from build123d import *

# Parameters (mm, degrees)
F0_W     = 60
F0_H     = 30
F1_DEPTH = 30
F2_W     = 30
F2_H     = 30
F3_DEPTH = 40
F3_TAPER = 7
F4_R     = 5.4270060884
F5_DEPTH = 40


with BuildPart() as f1:
    # F0 (on Front) → F1 (new body)
    with BuildSketch(Plane.XZ):
        with Locations((-30, -15)):
            Rectangle(F0_W, F0_H)
    extrude(amount=F1_DEPTH)

    # F2 (on face) → F3 (join)
    with BuildSketch(Plane.XY):
        with Locations((-15, -15)):
            Rectangle(F2_W, F2_H)
    extrude(amount=F3_DEPTH, taper=F3_TAPER)

    # F4 (on face) → F5 (cut)
    with BuildSketch(Plane.XY.offset(40)):
        with Locations((-14.5341902971, -15)):
            Circle(F4_R)
    extrude(amount=-F5_DEPTH, mode=Mode.SUBTRACT)


solid = f1.part
Geometry check sheet. Reference: the model listing, model coordinates, mm. A direction names the side the tool comes from. Give positions to 0.01 mm unless a question says otherwise; leave off trailing zeros. Order: outer loops, then holes, each group sorted by start corner. A loop starts at its lowest first (then second) coordinate and runs counter-clockwise, first axis right, second up.
1) Cross-section at C-C (x = -3.5). Record the boundary of the cut face in (y, z), then the cut area to 3 significant figures.
Results are:
outline: (-30, -30) - (0, -30) - (0, 0) - (-3.5, 28.51) - (-26.5, 28.51) - (-30, 0) - close
area: 1,660 mm2
2) Material ranges on probe 1 along Y at (x, z) = (-19, 37); probe 2 along X at (y, z) = (-18, 33.5); probe 3 along Y at (x, z) = (-11, 36), recorded low to high.
Results are:
probe 1: y = -25.46 to -18.08, -11.92 to -4.54
probe 2: x = -25.89 to -19.06, -10.01 to -4.11
probe 3: y = -25.58 to -19.12, -10.88 to -4.42
3) Cross-section at A-A (z = 16). Record the boundary of the cut face in (x, y), then the cut area to 3 significant figures.
Results are:
outline: (-28.04, -28.04) - (-1.96, -28.04) - (-1.96, -1.96) - (-28.04, -1.96) - close; hole circle Ø10.85 at (-14.53, -15)
area: 587 mm2
4) Tool access check on faces 4 (the flat face through (-30, -30, -15)), 5 (the flat face through (-45, -15, 0)), 6 (the cylindrical face through (-19.956, -14.761, 20.28)). Record the directions out of +Z, -Z, +X, -X, +Y, -Y that give a thin tool (end or side, any length) a straight path to the whole face; none if there is none.
Results are:
face 4: +Z, -Z, +X, -X, -Y
face 5: +Z, -X, +Y, -Y
face 6: +Z
5) Gauge pin test, flat ends, axial feed: pin 1 (10 mm diameter, centred on y = -11.5, z = 28, fed in from +X); pin 2 (1 mm diameter, centred on y = -17.5, z = 27, fed in from +X); pin 3 (5.5 mm diameter, centred on x = -13.5, y = -16.5, fed in from +Z). Record the tip position at first contact, or that the pin passes through.
Results are:
pin 1: stops at x = -2.82
pin 2: stops at x = -3.25
pin 3: stops at z = 0
6) Cross-section at B-B (y = -21.5). Record the boundary of the cut face in (x, z).
Results are:
outline: (-60, -30) - (0, -30) - (0, 0) - (-4.91, 40) - (-25.09, 40) - (-30, 0) - (-60, 0) - close
7) Draft check along Y on faces 1 (the flat face through (-27.58, -15.21, 19.72)), 2 (the flat face through (-15, -15, 0)), 3 (the flat face through (-15.21, -2.42, 19.72)). Enter one of: released by +Y, released by -Y, zero draft, split by the parting line, or undercut.
Results are:
face 1: zero draft
face 2: undercut
face 3: released by +Y
8) Cross-section at D-D (y = -2.25). Record the boundary of the cut face in (x, z).
Results are:
outline: (-60, -30) - (0, -30) - (0, 0) - (-2.25, 18.32) - (-27.75, 18.32) - (-30, 0) - (-60, 0) - close
